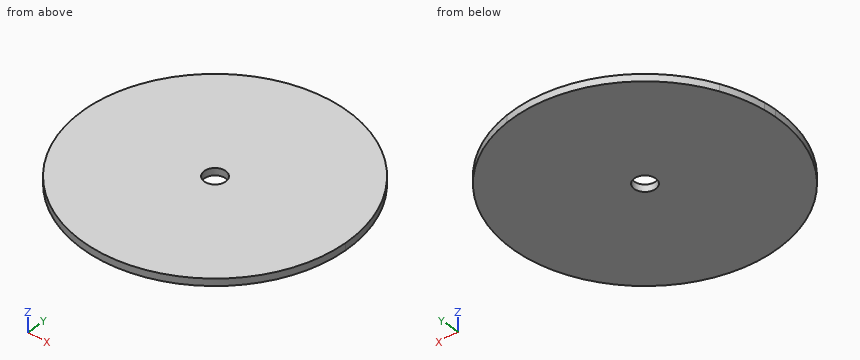
from build123d import *

# Parameters (mm, degrees)
F1_DEPTH = 3.175


# Not quite as in the source:
# - a length typed as a fraction of an inch, garbled in the dataset ("3 / 203.2 mm" for 3/8 in), is restored
# - a feature names something its author has since deleted; it is built from what else it names


with BuildPart() as f1:
    # F0 (on Top) → F1 (new body)
    with BuildSketch(Plane.XY):
        with BuildLine():
            Line((-12.6873488794, 5.5338457858), (-12.6873488794, -31.1003914823))
            ThreePointArc((-12.6873488794, -31.1003914823), (16.4381102813, -21.6348312874), (34.4341148999, 3.1448583573))
            ThreePointArc((34.4341148999, 3.1448583573), (36.2459189148, 10.6981520789), (36.8548431206, 18.4418005177))
            ThreePointArc((36.8548431206, 18.4418005177), (36.6946973558, 22.4220389265), (36.2152954077, 26.3765449929))
            ThreePointArc((36.2152954077, 26.3765449929), (10.5526750719, 26.4063777177), (-12.6873488794, 15.5218814393))
            Line((-12.6873488794, 15.5218814393), (-12.6873488794, 5.5338457858))
        make_face()
        with BuildLine():
            ThreePointArc((34.4341148999, 3.1448583573), (44.4839092315, -60.225850643), (-12.6873488794, -31.1003914823))
            Line((-12.6873488794, -31.1003914823), (-35.5892182517, -31.1003914823))
            ThreePointArc((-35.5892182517, -31.1003914823), (23.3171511206, -90.0067608546), (82.2235204929, -31.1003914823))
            ThreePointArc((82.2235204929, -31.1003914823), (69.3048842905, 5.7111386477), (36.2152954077, 26.3765449929))
            ThreePointArc((36.2152954077, 26.3765449929), (36.6946973558, 22.4220389265), (36.8548431206, 18.4418005177))
            ThreePointArc((36.8548431206, 18.4418005177), (36.2459189148, 10.6981520789), (34.4341148999, 3.1448583573))
        make_face()
        with BuildLine():
            ThreePointArc((34.4341148999, 3.1448583573), (16.4381102813, -21.6348312874), (-12.6873488794, -31.1003914823))
            ThreePointArc((-12.6873488794, -31.1003914823), (44.4839092315, -60.225850643), (34.4341148999, 3.1448583573))
        make_face()
        with BuildLine():
            ThreePointArc((28.0796511206, -31.1003914823), (23.3171511206, -35.8628914823), (18.5546511206, -31.1003914823))
            ThreePointArc((18.5546511206, -31.1003914823), (23.3171511206, -26.3378914823), (28.0796511206, -31.1003914823))
        make_face(mode=Mode.SUBTRACT)
        with BuildLine():
            ThreePointArc((-35.3338578497, -25.6213861535), (-24.3372830845, -29.7111622279), (-12.6873488794, -31.1003914823))
            Line((-12.6873488794, -31.1003914823), (-12.6873488794, 5.5338457858))
            Line((-12.6873488794, 5.5338457858), (-30.6664273508, -7.5263886814))
            ThreePointArc((-30.6664273508, -7.5263886814), (-33.7222633699, -16.3876233128), (-35.3338578497, -25.6213861535))
        make_face()
        with BuildLine():
            Line((-35.5892182517, -31.1003914823), (-12.6873488794, -31.1003914823))
            ThreePointArc((-12.6873488794, -31.1003914823), (-24.3372830845, -29.7111622279), (-35.3338578497, -25.6213861535))
            ThreePointArc((-35.3338578497, -25.6213861535), (-35.5253435202, -28.3579150318), (-35.5892182517, -31.1003914823))
        make_face()
        with BuildLine():
            Line((-30.6664273508, -7.5263886814), (-12.6873488794, 5.5338457858))
            Line((-12.6873488794, 5.5338457858), (-12.6873488794, 15.5218814393))
            ThreePointArc((-12.6873488794, 15.5218814393), (-23.129261611, 5.1306876763), (-30.6664273508, -7.5263886814))
        make_face()
    extrude(amount=F1_DEPTH)


solid = f1.part
Source: CAD feature listing. Evaluate the final solid. Frame: model axes, mm. Round coordinates to 2 decimals unless told otherwise and drop trailing zeros. Loops run counter-clockwise (first coordinate to the right, second up) from the corner with the lowest first, then second, coordinate; pieces in that order, holes last. Notation, with made-up numbers: (82, -23) -> (134, -23) arc R20 cw to (134, 7) -> close; hole circle Ø1 at (75.25, 40). An arc over 180 degrees is marked (long way). Answer as a JSON object with one key per item and string values. Group by question number.
Q1. Section query B-B (y = -77). Output: boundary loops of the cut face in (x, z) (1 decimal).
Q2. Ray query, line 1 (X direction, y = -28, z = 0.95); line 2 (X direction, y = -49, z = 1.75); line 3 (Y direction, x = 59.5, z = 2.45). Return the intervals inside material, ascending. Write a range as from..to.
Q3. Section query C-C (x = -27). Output: boundary loops of the cut face in (y, z) (3 decimals).
Q4. Contact query for a flat-ended pin moving along its axis: P1, Ø1, axis at y = -22.5, z = 2, coming from the -X side. Output: stop coordinate, or through.
Q5. Section query A-A (z = 0.8). Output: boundary loops of the cut face in (x, y) (1 decimal), plus the area to 3 significant figures.
Completed:
{
 "1": {"outline": "(-13.6, 0) -> (60.2, 0) -> (60.2, 3.2) -> (-13.6, 3.2) -> close"},
 "2": {"line 1": "-35.51..19.7, 26.93..82.14", "line 2": "-32.8..79.44", "line 3": "-77.58..15.38"},
 "3": {"outline": "(-61.73, 0) -> (-0.471, 0) -> (-0.471, 3.175) -> (-61.73, 3.175) -> close"},
 "4": {"P1": "x = -35.03"},
 "5": {"outline": "circle Ø117.8 at (23.3, -31.1); hole circle Ø9.5 at (23.3, -31.1)", "area": "10,800 mm²"}
}
